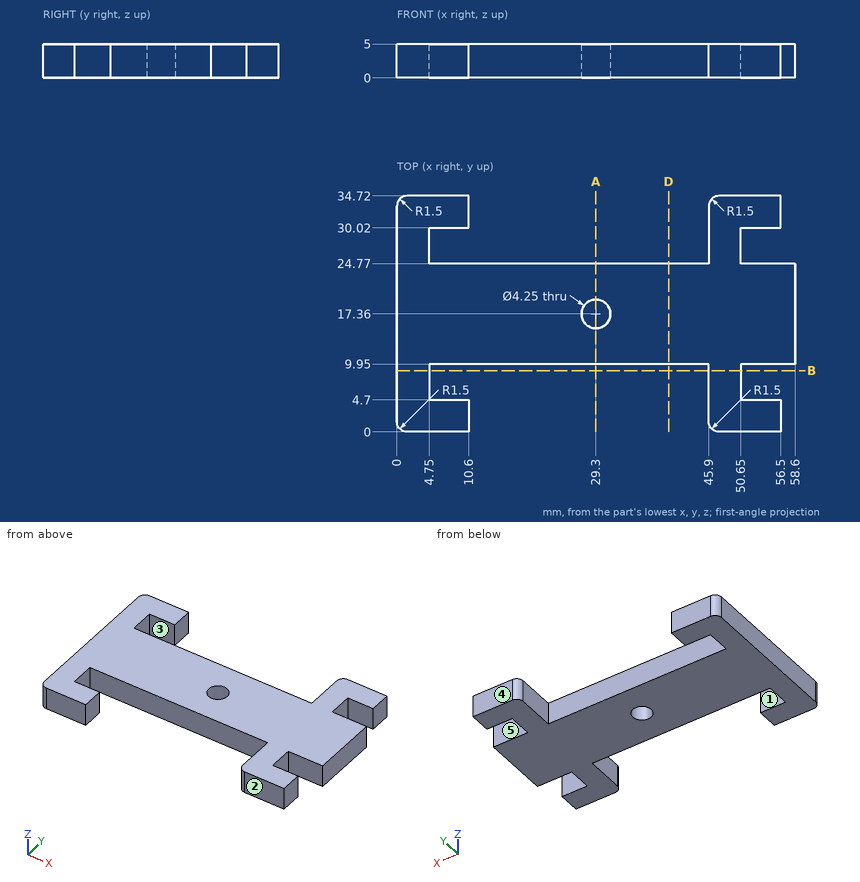
Here's the drawing with two shaded views (mm, measured from the low corner). I have some questions. A direction names the side the tool comes from. Coordinates: 2 decimals unless noted, no trailing zeros. Loops run counter-clockwise (first coordinate to the right, second up) from the corner with the lowest first, then second, coordinate; pieces in that order, holes last. Notation, with made-up numbers: (4.25, -26) -> (21.25, -26) arc R13 cw to (21.25, -14) -> close; hole circle Ø6 at (73, 37.5). An arc over 180 degrees is marked (long way). Put each result on its own line as item: value. Start each with the question number.
Q1. Thinking about a two-plate mould opening in X: for the marked faces 1 and 2, which applies, pulls with the +X half, pulls with the -X half, needs draft (parallel to the pull), parting line crosses it, or undercut?
Q2. I want a section at B-B (y = 9). Write out the boundary of the cut face in (x, z).
Q3. I want a section at D-D (x = 40). Write out the boundary of the cut face in (y, z), plus the area to 3 significant figures.
Q4. I want a section at A-A (x = 29.3). Write out the boundary of the cut face in (y, z) (3 decimals), plus the area to 4 significant figures.
Q5. For the marked faces 3, 4 and 5, which set-ups out of +Z, -Z, +X, -X, +Y, -Y let a thin tool reach every point of the face, with its end or its side?
Q6. If I drill on line 1 (Y direction, x = 54, z = 1.9); line 2 (X direction, y = 17.36, z = 2.8) (3 decimals); line 3 (Y direction, x = 29.3, z = 1.7) (3 decimals), over which ranges is the centre line in solid material (lowest first)? Write a range as [from, to].
Q7. I'm going to push flat-ended pins straight in: P1, Ø2.5, axis at y = 2, z = 3, coming from the +X side; P2, Ø1.5, axis at x = 33.5, z = 2, coming from the -Y side; P3, Ø1.5, axis at y = 27.5, z = 1.5, coming from the +X side. Where does each tip first touch, or does it pass through?
Taken from the geometry:
1. face 1: undercut
1. face 2: needs draft
2. outline: (0, 0) -> (4.75, 0) -> (4.75, 5) -> (0, 5) -> close; (45.9, 0) -> (50.65, 0) -> (50.65, 5) -> (45.9, 5) -> close
3. outline: (9.95, 0) -> (24.77, 0) -> (24.77, 5) -> (9.95, 5) -> close
3. area: 74.1 mm2
4. outline: (9.95, 0) -> (15.235, 0) -> (15.235, 5) -> (9.95, 5) -> close; (19.485, 0) -> (24.77, 0) -> (24.77, 5) -> (19.485, 5) -> close
4. area: 52.85 mm2
5. face 3: +Z, -Z
5. face 4: +Z, -Z, +X, -X, +Y
5. face 5: +Z, -Z, +X
6. line 1: y = [0, 4.7], [9.95, 24.77], [30.02, 34.72]
6. line 2: x = [0, 27.175], [31.425, 58.6]
6. line 3: y = [9.95, 15.235], [19.485, 24.77]
7. P1: stops at x = 56.5
7. P2: stops at y = 9.95
7. P3: stops at x = 50.65
